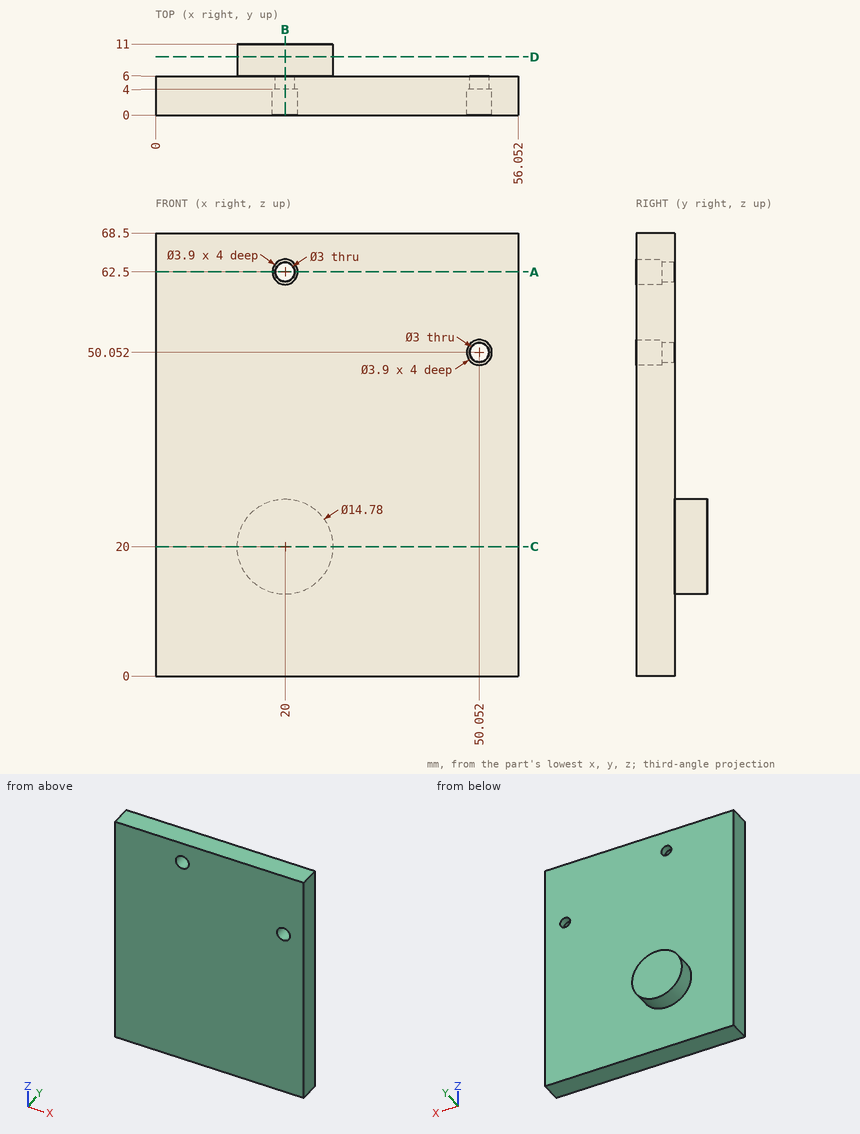
Geometry: see drawing. Coordinates: mm, zero at the bounding-box minimum. Give positions to 0.01 mm unless a question says otherwise; leave off trailing zeros. Order: outer loops, then holes, each group sorted by start corner. A loop starts at its lowest first (then second) coordinate and runs counter-clockwise, first axis right, second up. Notation, with made-up numbers: M 3.25,56.25 L 39.25,56.25 A12 ccw 39.25,78.25 Z; hole C -28,87.5 d3. An arc over 180 degrees is marked long. Answer as CSV lines item,"result". Start each with the question number.
1) First-contact query: P1, Ø3.5, axis at x = 20, z = 62.5, coming from the +Y side; P2, Ø1, axis at x = 17, y = 8, coming from the +Z side. Flat tips, straight axial feed; report the tip coordinate or a pass-through.
2) Cut plane A-A (z = 62.5). Output: boundary loops of the cut face in (x, y).
3) Cut plane C-C (z = 20). Output: boundary loops of the cut face in (x, y).
4) Cut plane D-D (y = 9). Output: boundary loops of the cut face in (x, z).
5) Line query: line 1 (Z direction, x = 20, y = 4.6); line 2 (X direction, y = 5.4, z = 62.5); line 3 (Y direction, x = 39, z = 12.5). Output: solid intervals per line, ascending. Write a range as from..to.
6) Cut plane B-B (x = 20). Output: boundary loops of the cut face in (y, z).
Findings below:
1,P1,"stops at y = 6"
1,P2,"stops at z = 26.95"
2,outline,"M 0,0 L 18.05,0 L 18.05,4 L 18.5,4 L 18.5,6 L 0,6 Z; M 21.5,4 L 21.95,4 L 21.95,0 L 56.05,0 L 56.05,6 L 21.5,6 Z"
3,outline,"M 0,0 L 56.05,0 L 56.05,6 L 27.39,6 L 27.39,11 L 12.61,11 L 12.61,6 L 0,6 Z"
4,outline,"C 20,20 d14.78"
5,line 1,"z = 0..61, 64..68.5"
5,line 2,"x = 0..18.5, 21.5..56.05"
5,line 3,"y = 0..6"
6,outline,"M 0,0 L 6,0 L 6,12.61 L 11,12.61 L 11,27.39 L 6,27.39 L 6,61 L 4,61 L 4,60.55 L 0,60.55 Z; M 0,64.45 L 4,64.45 L 4,64 L 6,64 L 6,68.5 L 0,68.5 Z"
